Check sheet for the modelled part. Datum: model origin and axes. Units: mm. A direction names the side the tool comes from. Round coordinates to 2 decimals unless told otherwise and drop trailing zeros. Order: outer loops, then holes, each group sorted by start corner. A loop starts at its lowest first (then second) coordinate and runs counter-clockwise, first axis right, second up. Notation, with made-up numbers: (-26.75, -32) -> (25.25, -32) arc R12 ccw to (25.25, -24) -> close; hole circle Ø4 at (74, 66.5). An arc over 180 degrees is marked (long way). Answer in a Markdown table with one row per item.
from build123d import *

# Parameters (mm, degrees)
BASPROSKE_W              = 8
BASPROSKE_H              = 30
TOOTHCUT_DEPTH           = 44.17406629
TEETHCUTS_COUNT          = 28
TEETHCUTS_ANGLE          = 347.142857143
BORSKE_R                 = 0.1
BORE_DEPTH               = 50.0000508
TAGLIO_ESTRUSIONE1_DEPTH = 30
SCHIZZO2_R               = 1.6
TAGLIO_ESTRUSIONE2_DEPTH = 10


with BuildPart() as part:
    # BasProSke → Base-Revolve (revolve)
    with BuildSketch(Plane(origin=(0, 0, 0), x_dir=(1, 0, 0), z_dir=(0, 1, 0)), mode=Mode.PRIVATE) as base_revolve_sk:
        with Locations((4, 15)):
            Rectangle(BASPROSKE_W, BASPROSKE_H)
    revolve(base_revolve_sk.sketch.rotate(Axis((-10, 0, 0), (1, 0, 0)), 180), axis=Axis((-10, 0, 0), (1, 0, 0)))

    # TooCutSke → ToothCut (cut, through all)
    with BuildSketch(Plane(origin=(0, 0, 0), x_dir=(0, 0, -1), z_dir=(1, 0, 0))):
        with BuildLine():
            ThreePointArc((0.928503763, 25.482089431), (0, 25.499), (-0.928503763, 25.482089431))
            ThreePointArc((-0.928503763, 25.482089431), (-1.618524429, 27.789411612), (-2.78585155, 29.895880591))
            ThreePointArc((-2.78585155, 29.895880591), (0, 30.0254), (2.78585155, 29.895880591))
            ThreePointArc((2.78585155, 29.895880591), (1.618524429, 27.789411612), (0.928503763, 25.482089431))
        make_face()
    toothcut = extrude(amount=TOOTHCUT_DEPTH, mode=Mode.SUBTRACT)

    # TeethCuts: ToothCut ×28 about axis
    teethcuts_axis = Axis((-10, 0, 0), (1, 0, 0))
    for i in range(1, TEETHCUTS_COUNT):
        add(toothcut.rotate(teethcuts_axis, i * TEETHCUTS_ANGLE / (TEETHCUTS_COUNT - 1)), mode=Mode.SUBTRACT)

    # BorSke → Bore (cut, symmetric)
    with BuildSketch(Plane(origin=(0, 0, 0), x_dir=(0, 0, -1), z_dir=(1, 0, 0))):
        with Locations(Location((0, 0, 0), (0, 0, 180))):
            Circle(BORSKE_R)
    extrude(amount=BORE_DEPTH, both=True, mode=Mode.SUBTRACT)

    # Schizzo1 → Taglio-Estrusione1 (cut)
    with BuildSketch(Plane(origin=(8, 0, 0), x_dir=(0, 0, -1), z_dir=(1, 0, 0))):
        with BuildLine():
            Line((-1.5, 2), (1.5, 2))
            ThreePointArc((1.5, 2), (0, -2.5), (-1.5, 2))
        make_face()
    extrude(amount=-TAGLIO_ESTRUSIONE1_DEPTH, mode=Mode.SUBTRACT)

    # Schizzo2 → Taglio-Estrusione2 (cut)
    with BuildSketch(Plane.ZY):
        with Locations((0, 8)):
            Circle(SCHIZZO2_R)
        with Locations((8, 0)):
            Circle(SCHIZZO2_R)
        with Locations((0, -8)):
            Circle(SCHIZZO2_R)
        with Locations((-8, 0)):
            Circle(SCHIZZO2_R)
    extrude(amount=-TAGLIO_ESTRUSIONE2_DEPTH, mode=Mode.SUBTRACT)


solid = part.part
Item 1: Mould release check, pull along Z, two halves, no side actions. Record for faces 1 (the cylindrical face through (3.94, 1.6, -27.74)), 2 (the cylindrical face through (3.944, 15.888, -19.944)): pulls with the +Z half, pulls with the -Z half, needs draft (parallel to the pull), parting line crosses it, or undercut.
Result sheet:
| item | result |
|---|---|
| face 1 | pulls with the -Z half |
| face 2 | undercut |
Item 2: Cross-section at C-C (x = 5). State how many separate pieces and enclosed holes the cut face has, and give its area (3 significant figures).
Result sheet:
| item | result |
|---|---|
| separate pieces | 1 |
| enclosed holes | 5 |
| area | 2,360 mm^2 |
Item 3: Set-up check for faces 3 (the cylindrical face through (3.94, -26.69, -7.73)), 4 (the cylindrical face through (3.94, -16.05, -22.69)), 5 (the cylindrical face through (3.94, 7.73, -26.69)), 6 (the cylindrical face through (3.944, 24.857, -5.687)): record each of +Z, -Z, +X, -X, +Y, -Y from which the full face is reachable in a straight line by a thin tool's end or side.
Result sheet:
| item | result |
|---|---|
| face 3 | +X, -X, -Y |
| face 4 | +X, -X |
| face 5 | -Z, +X, -X |
| face 6 | +X, -X, +Y |
Item 4: Cross-section at A-A (z = 8). Record the boundary of the cut face in (x, y), and give its area (3 significant figures).
Result sheet:
| item | result |
|---|---|
| outline | (0, -27.05) -> (8, -27.05) -> (8, -1.6) -> (0, -1.6) -> close; (0, 1.6) -> (8, 1.6) -> (8, 27.05) -> (0, 27.05) -> close |
| area | 407 mm^2 |
Item 5: Depth check by flat-ended pin: P1, Ø3, axis at x = 4.5, z = 7, coming from the +Y side; P2, Ø1, axis at x = 7, y = -5.5, coming from the -Z side; P3, Ø1.5, axis at x = 3.5, z = -23, coming from the -Y side. Enter the tip coordinate at first touch or a pass-through.
Result sheet:
| item | result |
|---|---|
| P1 | stops at y = 27.65 |
| P2 | stops at z = -25 |
| P3 | stops at y = -16.3 |
Item 6: Cross-section at D-D (z = 18). Record the boundary of the cut face in (x, y).
Result sheet:
| item | result |
|---|---|
| outline | (0, -20.37) -> (8, -20.37) -> (8, 20.37) -> (0, 20.37) -> close |
Item 7: Scan lines: line 1 (Y direction, x = 4, z = 0); line 2 (Z direction, x = 6, y = 27.5); line 3 (Y direction, x = 1.5, z = -15.5). Record each from-to range of solid material in increasing order. Write a range as [from, to].
Result sheet:
| item | result |
|---|---|
| line 1 | y = [-25.5, -9.6], [-6.4, -2.5], [2, 6.4], [9.6, 25.5] |
| line 2 | z = [-10.55, -8.37], [-4.6, -1.5], [1.5, 4.6], [8.37, 10.55] |
| line 3 | y = [-25.69, -21.19], [-20.25, 20.25], [21.19, 25.69] |
